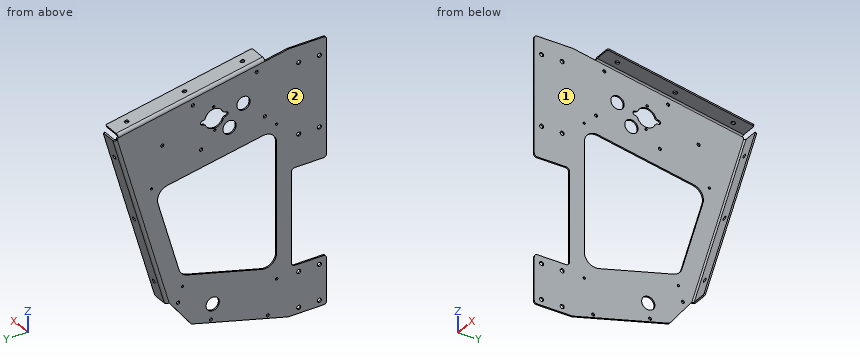
from build123d import *

# Parameters (mm, degrees)
SKETCH1_R                            = 14.2875
SKETCH1_R_2                          = 3.37312
BOSS_EXTRUDE1_DEPTH                  = 3.175
EDGE_FLANGE1_DEPTH                   = 399.923481586
SKETCH5_R                            = 14.2875
SKETCH5_R_2                          = 3.37312
SKETCH5_R_3                          = 2.5527
SKETCH5_R_4                          = 3.3734375
CUT_EXTRUDE1_DEPTH                   = 612.935699735
EDGE_FLANGE2_DEPTH                   = 371.853711622
F_11_32_0_34375_DIAMETER_HOLE3_D     = 8.73125
F_1_4_0_25_DIAMETER_HOLE1_D          = 6.35
F_17_64_0_26563_DIAMETER_HOLE2_D     = 6.747002
F_11_32_0_34375_DIAMETER_HOLE1_D     = 8.73125
F_11_32_0_34375_DIAMETER_HOLE2_D     = 8.73125
F_11_32_0_34375_DIAMETER_HOLE2_DEPTH = 3.175
F_10_0_1935_DIAMETER_HOLE1_D         = 4.9149
CUT_EXTRUDE2_START                   = -50.8
CUT_EXTRUDE2_DEPTH                   = 50.8
FILLET1_R                            = 3.175


# Sheet-metal steps are written as plain solids
with BuildPart() as part:
    # Sketch1 → Boss-Extrude1 (new body)
    with BuildSketch(Plane(origin=(0, 0, 0), x_dir=(0, 0, -1), z_dir=(1, 0, 0))):
        with BuildLine():
            Line((397.810445414, 0), (306.604125414, 0))
            ThreePointArc((306.604125414, 0), (301.552731346, 2.092355932), (299.460375414, 7.14375))
            Line((299.460375414, 7.14375), (299.460375414, 68.80225))
            ThreePointArc((299.460375414, 68.80225), (297.368019482, 73.853644068), (292.316625414, 75.946))
            Line((292.316625414, 75.946), (98.641625414, 75.946))
            ThreePointArc((98.641625414, 75.946), (93.590231346, 73.853644068), (91.497875414, 68.80225))
            Line((91.497875414, 68.80225), (91.497875414, 7.14375))
            ThreePointArc((91.497875414, 7.14375), (89.405519482, 2.092355932), (84.354125414, 0))
            Line((84.354125414, 0), (-158.75, 0))
            ThreePointArc((-158.75, 0), (-163.240128061, 1.859871939), (-165.1, 6.35))
            Line((-165.1, 6.35), (-165.1, 81.994446987))
            ThreePointArc((-165.1, 81.994446987), (-165.075836333, 82.547885953), (-165.003529232, 83.097112915))
            Line((-165.003529232, 83.097112915), (-100.43180985, 449.301531106))
            ThreePointArc((-100.43180985, 449.301531106), (-98.981933252, 451.446245541), (-96.4172045, 451.798536022))
            Line((-96.4172045, 451.798536022), (287.551897257, 339.965982534))
            Line((287.551897257, 339.965982534), (347.134178996, 293.415202216))
            ThreePointArc((347.134178996, 293.415202216), (348.525632464, 291.907463008), (349.363704269, 290.034749489))
            Line((349.363704269, 290.034749489), (403.949421055, 83.617862545))
            ThreePointArc((403.949421055, 83.617862545), (404.107468334, 82.812983692), (404.160445414, 81.994446987))
            Line((404.160445414, 81.994446987), (404.160445414, 6.35))
            ThreePointArc((404.160445414, 6.35), (402.300573474, 1.859871939), (397.810445414, 0))
        make_face()
        with Locations((-82.55, 179.578)):
            Circle(SKETCH1_R, mode=Mode.SUBTRACT)
        with Locations((-51.675354011, 354.676818486)):
            Circle(SKETCH1_R_2, mode=Mode.SUBTRACT)
        with Locations((321.610445414, 245.95582)):
            Circle(SKETCH1_R, mode=Mode.SUBTRACT)
        with BuildLine():
            Line((25.362018074, 107.95), (259.432488996, 107.95))
            ThreePointArc((259.432488996, 107.95), (279.55833085, 117.854500987), (283.988391562, 139.843662232))
            Line((283.988391562, 139.843662232), (241.393515847, 300.916964234))
            ThreePointArc((241.393515847, 300.916964234), (235.020226293, 312.158932355), (223.940339151, 318.810005043))
            Line((223.940339151, 318.810005043), (68.8320461, 363.985922583))
            ThreePointArc((68.8320461, 363.985922583), (48.314216085, 361.16759873), (36.715203303, 344.009883255))
            Line((36.715203303, 344.009883255), (0.347901148, 137.760663713))
            ThreePointArc((0.347901148, 137.760663713), (5.904489219, 117.023194714), (25.362018074, 107.95))
        make_face(mode=Mode.SUBTRACT)
    extrude(amount=-BOSS_EXTRUDE1_DEPTH)

    # Edge-Flange1 section (across the edge) → Edge-Flange1 (add)
    with BuildSketch(Plane(origin=(0, 343.014320414, -288.439737991), x_dir=(3.4914813388431334e-15, -0.9601064189437505, 0.27963487676434007), z_dir=(0, 0.27963487676434007, 0.9601064189437505))):
        with BuildLine():
            Line((-3.175, 3.175), (-3.175, 34.925))
            Line((-3.175, 34.925), (0, 34.925))
            Line((0, 34.925), (0, 3.175))
            ThreePointArc((0, 3.175), (0.92993597, 0.92993597), (3.175, 0))
            Line((3.175, 0), (3.175, -3.175))
            ThreePointArc((3.175, -3.175), (-1.315128061, -1.315128061), (-3.175, 3.175))
        make_face()
    extrude(amount=EDGE_FLANGE1_DEPTH)

    # Sketch5 → Cut-Extrude1 (cut, through all)
    with BuildSketch(Plane.ZY.offset(3.175)):
        with Locations(Location((82.55, 179.578, 0), (0, 0, 180))):
            Circle(SKETCH5_R)
        with Locations(Location((51.675354011, 354.676818486, 0), (0, 0, 180))):
            Circle(SKETCH5_R_2)
        with Locations(Location((-321.610445414, 245.95582, 0), (0, 0, 180))):
            Circle(SKETCH5_R)
        with Locations((96.823649998, 243.734949129)):
            Circle(SKETCH5_R_3)
        with Locations((46.08261916, 241.287953106)):
            Circle(SKETCH5_R_3)
        with Locations((41.572725009, 209.603038456)):
            Circle(SKETCH5_R)
        with Locations((114.900475932, 288.654874532)):
            Circle(SKETCH5_R_4)
        with Locations((14.844008226, 271.012219681)):
            Circle(SKETCH5_R_4)
        with Locations((39.102658646, 133.434576585)):
            Circle(SKETCH5_R_4)
        with Locations((139.159126352, 151.077231436)):
            Circle(SKETCH5_R_4)
        with BuildLine():
            Line((65.865907916, 267.671524878), (65.896371611, 267.039828185))
            ThreePointArc((65.896371611, 267.039828185), (65.022940965, 263.507443035), (62.353599656, 261.034541314))
            ThreePointArc((62.353599656, 261.034541314), (50.839590801, 241.517358984), (64.178240374, 223.19870091))
            ThreePointArc((64.178240374, 223.19870091), (67.073153395, 220.994136431), (68.282440243, 217.562190734))
            Line((68.282440243, 217.562190734), (68.312903938, 216.930494041))
            ThreePointArc((68.312903938, 216.930494041), (72.887074248, 212.777207047), (77.040361242, 217.351377357))
            Line((77.040361242, 217.351377357), (77.009897547, 217.98307405))
            ThreePointArc((77.009897547, 217.98307405), (77.883328193, 221.5154592), (80.552669502, 223.988360921))
            ThreePointArc((80.552669502, 223.988360921), (92.066678357, 243.505543251), (78.728028784, 261.824201325))
            ThreePointArc((78.728028784, 261.824201325), (75.833115763, 264.028765804), (74.623828915, 267.460711501))
            Line((74.623828915, 267.460711501), (74.59336522, 268.092408194))
            ThreePointArc((74.59336522, 268.092408194), (70.01919491, 272.245695188), (65.865907916, 267.671524878))
        make_face()
    extrude(amount=-CUT_EXTRUDE1_DEPTH, mode=Mode.SUBTRACT)

    # Edge-Flange2 section (across the edge) → Edge-Flange2 (add)
    with BuildSketch(Plane(origin=(0, 449.85286407, 103.558574466), x_dir=(3.4914813388431334e-15, -0.17364817766692356, -0.9848077530122094), z_dir=(0, -0.9848077530122094, 0.17364817766692356))):
        with BuildLine():
            Line((-3.175, 3.175), (-3.175, 38.1))
            Line((-3.175, 38.1), (0, 38.1))
            Line((0, 38.1), (0, 3.175))
            ThreePointArc((0, 3.175), (0.92993597, 0.92993597), (3.175, 0))
            Line((3.175, 0), (3.175, -3.175))
            ThreePointArc((3.175, -3.175), (-1.315128061, -1.315128061), (-3.175, 3.175))
        make_face()
    extrude(amount=EDGE_FLANGE2_DEPTH)

    # 11/32 (0.34375) Diameter Hole3 (through all)
    with Locations(Plane(origin=(0, 0, 0), x_dir=(0, 0, -1), z_dir=(1, 0, 0))):
        with Locations((-129.221774586, 15.875), (-129.221774586, 60.325), (23.178225414, 15.875), (23.178225414, 60.325), (315.278225414, 60.325), (315.278225414, 15.875), (391.478225414, 15.875), (391.478225414, 60.325)):
            Hole(F_11_32_0_34375_DIAMETER_HOLE3_D / 2)

    # 1/4 (0.25) Diameter Hole1 (through all)
    with Locations(Plane(origin=(0, 0, 0), x_dir=(0, 0, -1), z_dir=(1, 0, 0))):
        with Locations((353.440683712, 249.779512828), (385.908994874, 127)):
            Hole(F_1_4_0_25_DIAMETER_HOLE1_D / 2)

    # 17/64 (0.26563) Diameter Hole2 (through all)
    with Locations(Plane.ZY.offset(3.175)):
        with Locations((-293.708669355, 320.539904842)):
            Hole(F_17_64_0_26563_DIAMETER_HOLE2_D / 2)

    # 11/32 (0.34375) Diameter Hole1 (through all)
    with Locations(Plane(origin=(0, 396.680507326, -115.53480176), x_dir=(1, 0, 0), z_dir=(-3.629989339958336e-15, 0.9601064189437505, -0.27963487676434007))):
        with Locations((19.05, 136.69059512), (19.05, -15.70940488), (19.05, -168.10940488)):
            Hole(F_11_32_0_34375_DIAMETER_HOLE1_D / 2)

    # 11/32 (0.34375) Diameter Hole2
    with Locations(Plane(origin=(0, 31.825615837, 180.492036493), x_dir=(1, 0, 0), z_dir=(-3.2076224383382817e-15, 0.17364817766692356, 0.9848077530122092))):
        with Locations((19.05, 391.508974703), (19.05, 264.508974703), (19.05, 137.508974703)):
            Hole(F_11_32_0_34375_DIAMETER_HOLE2_D / 2, depth=F_11_32_0_34375_DIAMETER_HOLE2_DEPTH)

    # #10 (0.1935) Diameter Hole1 (through all)
    with Locations(Plane.ZY.offset(3.175)):
        with Locations((-262.310998074, 311.15), (-314.845818074, 107.95), (14.185781926, 107.95), (-32.555298074, 377.825)):
            Hole(F_10_0_1935_DIAMETER_HOLE1_D / 2)

    # Sketch31 → Cut-Extrude2 (cut)
    with BuildSketch(Plane(origin=(0, 52.374163006, -9.23497803), x_dir=(1, 0, 0), z_dir=(-2.784783301719586e-15, -0.9848077530122092, 0.1736481776669235)).offset(CUT_EXTRUDE2_START)):
        with BuildLine():
            Line((3.175, 180.101417089), (38.1, 180.101417089))
            Line((38.1, 180.101417089), (38.1, 183.276417089))
            Line((38.1, 183.276417089), (3.175, 183.276417089))
            ThreePointArc((3.175, 183.276417089), (-1.315128061, 181.416545149), (-3.175, 176.926417089))
            Line((-3.175, 176.926417089), (0, 176.926417089))
            ThreePointArc((0, 176.926417089), (0.92993597, 179.171481119), (3.175, 180.101417089))
        make_face()
    extrude(amount=CUT_EXTRUDE2_DEPTH, mode=Mode.SUBTRACT)

    # Fillet1
    fillet1_edges = [part.edges().sort_by_distance(p)[0] for p in [
        (38.1, 450.128530552, 105.121956774),
        (38.1, 133.952346214, 160.87234873),
        (34.925, 344.538489354, -288.883658358),
        (34.925, 456.371042842, 95.0854434),
    ]]
    fillet(fillet1_edges, radius=FILLET1_R)


solid = part.part
Input: part model. Units: mm. Frame: model coordinates. Face numbers are marked on the shaded views. A direction names the side the tool comes from. Give positions to 0.01 mm unless a question says otherwise; leave off trailing zeros.
Q1. Set-up query: the marked faces 1 and 2. Return all of +Z, -Z, +X, -X, +Y, -Y with unobstructed straight access to the full face (end or side cutting, diameter ignored); none if empty.
Q2. First-contact query: P1, Ø3, axis at y = 311.15, z = -262.31, coming from the -X side; P2, Ø6, axis at x = 29.5, y = 207, coming from the -Z side; P3, Ø2, axis at x = 26.5, z = -101.5, coming from the -Y side; P4, Ø1, axis at x = -1.5, z = -167, coming from the -Y side. Flat tips, straight axial feed; report the tip coordinate or a pass-through.
Q3. Material intervals for probe 1 along Z at (x, y) = (-0.5, 202.5); probe 2 along X at (y, z) = (100, -224) (3 decimals); probe 3 along Y at (x, z) = (20, -69), sorted ascending.
Filled in:
1. face 1: +X, -Y
1. face 2: +Z, -Z, -X, +Y, -Y
2. P1: passes through
2. P2: stops at z = 145.85
2. P3: stops at y = 397.17
2. P4: stops at y = 75.95
3. probe 1: z = -372.51 to -267.42, -11.76 to 29.18, 53.97 to 149.21
3. probe 2: x = -3.175 to 0
3. probe 3: y = 406.93 to 410.23
